from build123d import *

# Parameters (mm, degrees)
SKETCH1_R               = 4.765
BOSS_EXTRUDE1_DEPTH     = 9.525
CHAMFER1_SIZE           = 0.76
SKETCH2_R               = 3.43
CUT_EXTRUDE1_DEPTH      = 5.765
CUT_EXTRUDE1_DEPTH_BACK = 5.765


with BuildPart() as part:
    # Sketch1 → Boss-Extrude1 (new body, symmetric)
    with BuildSketch(Plane.XY):
        Circle(SKETCH1_R)
    extrude(amount=BOSS_EXTRUDE1_DEPTH, both=True)

    # Chamfer1
    chamfer1_edges = [part.edges().sort_by_distance(p)[0] for p in [
        (-4.765, 0, -9.525),
        (-4.765, 0, 9.525),
    ]]
    chamfer(chamfer1_edges, length=CHAMFER1_SIZE)

    # Sketch2 → Cut-Extrude1 (cut, two sides)
    with BuildSketch(Plane(origin=(0, 0, 0), x_dir=(1, 0, 0), z_dir=(0, 1, 0))) as cut_extrude1_sk:
        with Locations((-0.25, 0)):
            Circle(SKETCH2_R)
    extrude(amount=CUT_EXTRUDE1_DEPTH, mode=Mode.SUBTRACT)
    extrude(cut_extrude1_sk.sketch, amount=-CUT_EXTRUDE1_DEPTH_BACK, mode=Mode.SUBTRACT)


solid = part.part
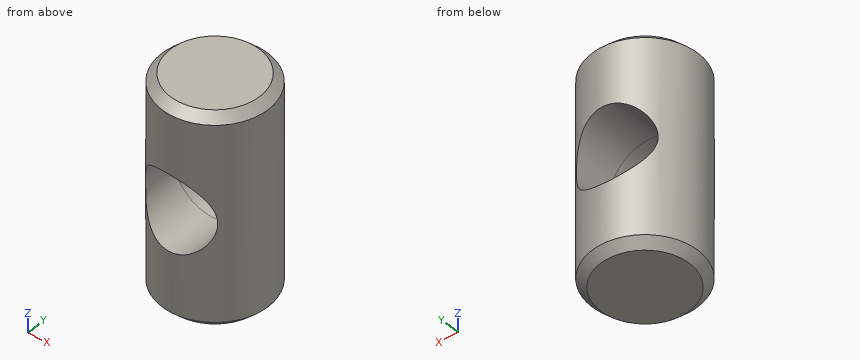
Check sheet for the modelled part. Datum: model origin and axes. Units: mm. Round coordinates to 2 decimals unless told otherwise and drop trailing zeros. Order: outer loops, then holes, each group sorted by start corner. A loop starts at its lowest first (then second) coordinate and runs counter-clockwise, first axis right, second up.
(1) Cross-section at C-C, the plane z = 0. Enter the section's corners in (x, y) (3 decimals).
(2) Cross-section at A-A, the plane x = 0. Enter the section's corners in (y, z) (3 decimals), and give its area (3 significant figures).
(3) Go/stop test with flat-tipped pins: P1, Ø1.5, axis at x = 2, z = -4.5, coming from the -Y side; P2, Ø1, axis at x = -1.5, z = 3.5, coming from the -Y side; P3, Ø4, axis at x = -0.25, z = 0, coming from the -Y side. Record where each tip stops, or that it passes through.
(4) Scan lines: probe 1 along Z at (x, y) = (-0.25, 3.05) (3 decimals); probe 2 along X at (y, z) = (-2.3, 0); probe 3 along X at (y, z) = (1.25, 0). Record each from-to range of solid material in increasing order.
(5) Cross-section at B-B, the plane z = 3. Enter the section's corners in (x, y) (3 decimals), and give its area (3 significant figures).
Check sheet entries:
1. outline: (-3.68, -3.027) - (-3.68, 3.027) arc R4.765 ccw to start; (3.18, -3.549) arc R4.765 ccw to (3.18, 3.549) - close
2. outline: (-4.765, -8.765) - (-4.005, -9.525) - (4.005, -9.525) - (4.765, -8.765) - (4.765, -3.421) - (-4.765, -3.421) - close; (-4.765, 3.421) - (4.765, 3.421) - (4.765, 8.765) - (4.005, 9.525) - (-4.005, 9.525) - (-4.765, 8.765) - close
2. area: 115 mm2
3. P1: stops at y = -4.6
3. P2: stops at y = -4.66
3. P3: passes through
4. probe 1: z = -9.525 to -3.43, 3.43 to 9.525
4. probe 2: x = -4.17 to -3.68, 3.18 to 4.17
4. probe 3: x = -4.6 to -3.68, 3.18 to 4.6
5. outline: (-1.913, -4.364) - (-1.913, 4.364) arc R4.765 ccw to start; (1.413, -4.551) arc R4.765 ccw to (1.413, 4.551) - close
5. area: 40.3 mm2
